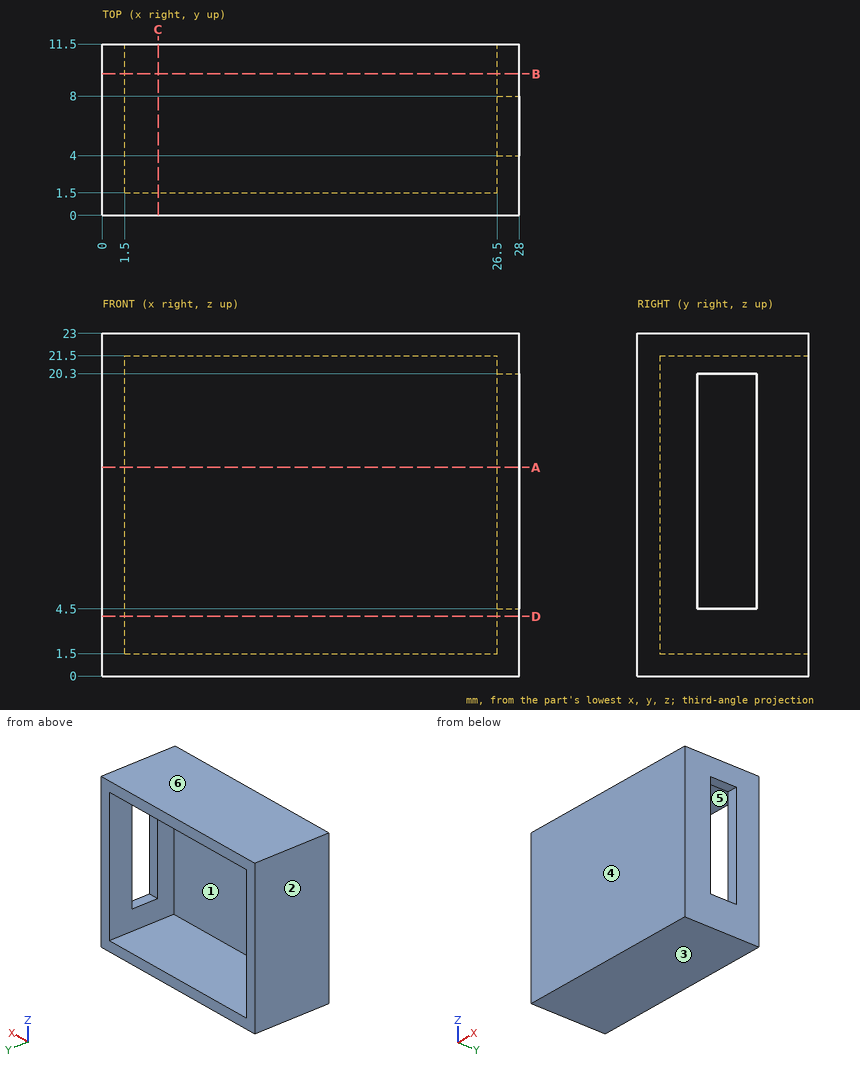
Geometry: see drawing. Coordinates: mm, zero at the bounding-box minimum. A direction names the side the tool comes from. Coordinates: 2 decimals unless noted, no trailing zeros. Order: outer loops, then holes, each group sorted by start corner. A loop starts at its lowest first (then second) coordinate and runs counter-clockwise, first axis right, second up. Notation, with made-up numbers: (41, 36.25) -> (70, 36.25) arc R24 ccw to (70, 52.25) -> close; hole circle Ø3 at (20.25, -4). An arc over 180 degrees is marked (long way). Write each question's results on one line, items separated by ' | '. Start each with the question number.
1) Material intervals for line 1 along Z through (x, y) = (22, 5); line 2 along X through (y, z) = (2, 16.5); line 3 along Y through (x, z) = (16, 11.25), sorted ascending.
2) Cut plane C-C, the plane x = 3.75. Output: boundary loops of the cut face in (y, z), and give its area (3 significant figures).
3) Mould query, pull axis Z, two halves, no side actions, for the marked faces 3, 4, 5 and 6. Classes: released by +Z, released by -Z, zero draft, split by the parting line, or undercut.
4) Cut plane A-A, the plane z = 14. Output: boundary loops of the cut face in (x, y).
5) Set-up query: the marked faces 1 and 2. Return all of +Z, -Z, +X, -X, +Y, -Y with unobstructed straight access to the full face (end or side cutting, diameter ignored); none if empty.
6) Cut plane B-B, the plane y = 9.5. Output: boundary loops of the cut face in (x, z).
7) Cut plane D-D, the plane z = 4. Output: boundary loops of the cut face in (x, y).
Checks:
1) line 1: 0 to 1.5, 21.5 to 23 | line 2: 0 to 1.5, 26.5 to 28 | line 3: 0 to 1.5
2) outline: (0, 0) -> (11.5, 0) -> (11.5, 1.5) -> (1.5, 1.5) -> (1.5, 21.5) -> (11.5, 21.5) -> (11.5, 23) -> (0, 23) -> close | area: 64.5 mm^2
3) face 3: released by -Z | face 4: zero draft | face 5: undercut | face 6: released by +Z
4) outline: (0, 0) -> (28, 0) -> (28, 4) -> (26.5, 4) -> (26.5, 1.5) -> (1.5, 1.5) -> (1.5, 11.5) -> (0, 11.5) -> close; (26.5, 8) -> (28, 8) -> (28, 11.5) -> (26.5, 11.5) -> close
5) face 1: +Y | face 2: +Z, -Z, -X, +Y, -Y
6) outline: (0, 0) -> (28, 0) -> (28, 23) -> (0, 23) -> close; hole (1.5, 1.5) -> (26.5, 1.5) -> (26.5, 21.5) -> (1.5, 21.5) -> close
7) outline: (0, 0) -> (28, 0) -> (28, 11.5) -> (26.5, 11.5) -> (26.5, 1.5) -> (1.5, 1.5) -> (1.5, 11.5) -> (0, 11.5) -> close
